Geometry check sheet. Reference: the model listing, model coordinates, mm. A direction names the side the tool comes from. Give positions to 0.01 mm unless a question says otherwise; leave off trailing zeros. Loops run counter-clockwise (first coordinate to the right, second up) from the corner with the lowest first, then second, coordinate; pieces in that order, holes last.
```python
from build123d import *

# Parameters (mm, degrees)
SKETCH1_W           = 25.4
SKETCH1_H           = 50.8
SKETCH1_W_2         = 20.32
SKETCH1_H_2         = 45.72
EXTRUDE_THIN1_DEPTH = 609.6
SKETCH2_R           = 1.5875
CUT_EXTRUDE1_DEPTH  = 51.8
LPATTERN1_COUNT     = 50
LPATTERN1_PITCH     = 25.4
CUT_EXTRUDE2_DEPTH  = 51.8
SKETCH5_R           = 1.5875
CUT_EXTRUDE3_DEPTH  = 26.4


with BuildPart() as part:
    # Sketch1 → Extrude-Thin1 (new body)
    with BuildSketch(Plane.XY):
        with Locations((12.7, 25.4)):
            Rectangle(SKETCH1_W, SKETCH1_H)
        with Locations((12.7, 25.4)):
            Rectangle(SKETCH1_W_2, SKETCH1_H_2, mode=Mode.SUBTRACT)
    extrude(amount=EXTRUDE_THIN1_DEPTH)

    # Sketch2 → Cut-Extrude1 (cut, through all)
    with BuildSketch(Plane(origin=(0, 50.8, 0), x_dir=(1, 0, 0), z_dir=(0, 1, 0))):
        with Locations((12.7, -596.9)):
            Circle(SKETCH2_R)
    cut_extrude1 = extrude(amount=-CUT_EXTRUDE1_DEPTH, mode=Mode.SUBTRACT)

    # LPattern1: Cut-Extrude1 ×50
    with Locations(*[(0, 0, -i * LPATTERN1_PITCH) for i in range(1, LPATTERN1_COUNT)]):
        add(cut_extrude1, mode=Mode.SUBTRACT)

    # Sketch4 → Cut-Extrude2 (cut, through all)
    with BuildSketch(Plane(origin=(0, 50.8, 0), x_dir=(1, 0, 0), z_dir=(0, 1, 0))):
        Polygon((0, -609.6), (25.4, -584.2), (25.4, -609.6), align=None)
        Polygon((0, 0), (25.4, 0), (25.4, -25.4), align=None)
    extrude(amount=-CUT_EXTRUDE2_DEPTH, mode=Mode.SUBTRACT)

    # Sketch5 → Cut-Extrude3 (cut, through all)
    with BuildSketch(Plane.ZY):
        with Locations((12.7, 12.7)):
            Circle(SKETCH5_R)
        with Locations((12.7, 38.1)):
            Circle(SKETCH5_R)
        with Locations((596.9, 38.1)):
            Circle(SKETCH5_R)
        with Locations((596.9, 12.7)):
            Circle(SKETCH5_R)
    extrude(amount=-CUT_EXTRUDE3_DEPTH, mode=Mode.SUBTRACT)


solid = part.part
```
1) Sectioned sample at B-B on z = 487. Enter the section's corners in (x, y).
2) Mould release check, pull along Y, two halves, no side actions. Record for faces 1 (the flat face through (13, 48.26, 301)), 2 (the flat face through (13, 0, 301)), 3 (the flat face through (0, 25, 301)), 4 (the flat face through (2.54, 25, 301)): +Y half, -Y half, draft (parallel to the pull), parting line (faces both ways), or undercut.
3) Scan lines: line 1 along Y through (x, z) = (12.5, 294); line 2 along X through (y, z) = (25, 433.5); line 3 along X through (y, z) = (1, 419). Record each from-to range of solid material in increasing order.
4) Sectioned sample at A-A on x = 18.75. Enter the section's corners in (y, z), plus the area to 3 significant figures.
5) Tool access check on faces 5 (the flat face through (25.4, 25, 301)), 6 (the flat face through (22.86, 25, 301)). Record the directions out of +Z, -Z, +X, -X, +Y, -Y that give a thin tool (end or side, any length) a straight path to the whole face; none if there is none.
6) Depth check by flat-ended pin: P1, Ø3, axis at x = 12.7, z = 368.3, coming from the +Y side. Enter the tip coordinate at first touch or a pass-through.
Determined:
1. outline: (0, 0) - (25.4, 0) - (25.4, 50.8) - (0, 50.8) - close; hole (2.54, 2.54) - (22.86, 2.54) - (22.86, 48.26) - (2.54, 48.26) - close
2. face 1: undercut
2. face 2: -Y half
2. face 3: draft
2. face 4: undercut
3. line 1: y = 0 to 2.54, 48.26 to 50.8
3. line 2: x = 0 to 2.54, 22.86 to 25.4
3. line 3: x = 0 to 11.12, 14.28 to 25.4
4. outline: (0, 18.75) - (2.54, 18.75) - (2.54, 590.85) - (0, 590.85) - close; (48.26, 18.75) - (50.8, 18.75) - (50.8, 590.85) - (48.26, 590.85) - close
4. area: 2,910 mm2
5. face 5: +Z, -Z, +X, +Y, -Y
5. face 6: +Z, -Z
6. P1: passes through
